from build123d import *

# Parameters (mm, degrees)
SKETCH_1_W             = 60
SKETCH_1_H             = 15
EXTRUDE_1_DEPTH        = 2
SKETCH_2_W             = 3
SKETCH_2_H             = 3
EXTRUDE_2_DEPTH        = 1
EXTRUDE_3_DEPTH        = 2
CUT_EXTRUDE_1_REACH    = 42.234
SKETCH_4_W             = 0.944409721
SKETCH_4_H             = 0.05
FILLET_1_R             = 0.1
FILLET_1_OF_MIRROR_2_R = 0.1
FILLET_2_R             = 0.2


# Read off the part's stored shape, not the designer's step: the mirror step
with BuildPart() as part:
    # Sketch 1 → Extrude 1 (new body)
    with BuildSketch(Plane.XY):
        Rectangle(SKETCH_1_W, SKETCH_1_H)
    extrude(amount=-EXTRUDE_1_DEPTH)

    # Sketch 2 → Extrude 2 (add)
    with BuildSketch(Plane.XY):
        with Locations((-7.5, 0)):
            Rectangle(SKETCH_2_W, SKETCH_2_H)
    extrude_2 = extrude(amount=EXTRUDE_2_DEPTH)

    # Sketch 3 → Extrude 3 (add, symmetric)
    with BuildSketch(Plane(origin=(0, 0, 0), x_dir=(1, 0, 0), z_dir=(0, 1, 0))):
        with BuildLine():
            Line((-9.45, -2.5), (-5.55, -2.5))
            Line((-5.55, -2.5), (-5.55, -1.555590279))
            ThreePointArc((-5.55, -1.555590279), (-5.719957697, -1.088161527), (-6, -0.677124344))
            Line((-6, -0.677124344), (-9, -0.677124344))
            ThreePointArc((-9, -0.677124344), (-9.280042303, -1.088161527), (-9.45, -1.555590279))
            Line((-9.45, -1.555590279), (-9.45, -2.5))
        make_face()
    extrude_3 = extrude(amount=EXTRUDE_3_DEPTH, both=True)

    # Sketch 4 → Cut-Extrude 1 (cut, up to next)
    with BuildSketch(Plane.ZY.offset(9.45), mode=Mode.PRIVATE) as cut_extrude_1_sk1:
        with BuildLine():
            Line((1.555590279, 1.95), (1.555590279, 2))
            Line((1.555590279, 2), (0.677124344, 2))
            Line((0.677124344, 2), (0.677124344, 1.5))
            ThreePointArc((0.677124344, 1.5), (1.088161527, 1.780042303), (1.555590279, 1.95))
        make_face()
    cut_extrude_1_tool1 = extrude(cut_extrude_1_sk1.sketch, amount=-CUT_EXTRUDE_1_REACH, mode=Mode.PRIVATE) & part.part
    # Sketch 4 → Cut-Extrude 1 (cut, up to next)
    with BuildSketch(Plane.ZY.offset(9.45), mode=Mode.PRIVATE) as cut_extrude_1_sk2:
        with Locations((2.02779514, 1.975)):
            Rectangle(SKETCH_4_W, SKETCH_4_H)
    cut_extrude_1_tool2 = extrude(cut_extrude_1_sk2.sketch, amount=-CUT_EXTRUDE_1_REACH, mode=Mode.PRIVATE) & part.part
    # Sketch 4 → Cut-Extrude 1 (cut, up to next)
    with BuildSketch(Plane.ZY.offset(9.45), mode=Mode.PRIVATE) as cut_extrude_1_sk3:
        with Locations((2.02779514, -1.975)):
            Rectangle(SKETCH_4_W, SKETCH_4_H)
    cut_extrude_1_tool3 = extrude(cut_extrude_1_sk3.sketch, amount=-CUT_EXTRUDE_1_REACH, mode=Mode.PRIVATE) & part.part
    # Sketch 4 → Cut-Extrude 1 (cut, up to next)
    with BuildSketch(Plane.ZY.offset(9.45), mode=Mode.PRIVATE) as cut_extrude_1_sk4:
        with BuildLine():
            Line((1.555590279, -2), (1.555590279, -1.95))
            ThreePointArc((1.555590279, -1.95), (1.088161527, -1.780042303), (0.677124344, -1.5))
            Line((0.677124344, -1.5), (0.677124344, -2))
            Line((0.677124344, -2), (1.555590279, -2))
        make_face()
    cut_extrude_1_tool4 = extrude(cut_extrude_1_sk4.sketch, amount=-CUT_EXTRUDE_1_REACH, mode=Mode.PRIVATE) & part.part
    cut_extrude_1_1 = cut_extrude_1_tool1.solids().sort_by_distance((-9.45, 1.849056, 0.974505))[0]
    add(cut_extrude_1_1, mode=Mode.SUBTRACT)
    cut_extrude_1_2 = cut_extrude_1_tool2.solids().sort_by_distance((-9.45, 1.975, 2.027795))[0]
    add(cut_extrude_1_2, mode=Mode.SUBTRACT)
    cut_extrude_1_3 = cut_extrude_1_tool3.solids().sort_by_distance((-9.45, -1.975, 2.027795))[0]
    add(cut_extrude_1_3, mode=Mode.SUBTRACT)
    cut_extrude_1_4 = cut_extrude_1_tool4.solids().sort_by_distance((-9.45, -1.849056, 0.974505))[0]
    add(cut_extrude_1_4, mode=Mode.SUBTRACT)
    cut_extrude_1 = cut_extrude_1_1 + cut_extrude_1_2 + cut_extrude_1_3 + cut_extrude_1_4  # Cut-Extrude 1 as one shape, for the pattern or mirror that repeats it

    # Fillet 1
    fillet_1_edges = [part.edges().sort_by_distance(p)[0] for p in [
        (-7.5, 1.95, 2.5),
        (-9.45, 0, 2.5),
        (-5.55, 0, 2.5),
        (-7.5, -1.95, 2.5),
    ]]
    fillet(fillet_1_edges, radius=FILLET_1_R)

    # Mirror 2: Extrude 2, Extrude 3, Cut-Extrude 1 across plane
    add(extrude_2.mirror(Plane(origin=(-15, 0, 0), x_dir=(0, 0, 1), z_dir=(1, 0, 0))))
    add(extrude_3.mirror(Plane(origin=(-15, 0, 0), x_dir=(0, 0, 1), z_dir=(1, 0, 0))))
    add(cut_extrude_1.mirror(Plane(origin=(-15, 0, 0), x_dir=(0, 0, 1), z_dir=(1, 0, 0))), mode=Mode.SUBTRACT)

    # Fillet 1 of Mirror 2
    fillet_1_of_mirror_2_edges = [part.edges().sort_by_distance(p)[0] for p in [
        (-22.5, 1.95, 2.5),
        (-20.55, 0, 2.5),
        (-24.45, 0, 2.5),
        (-22.5, -1.95, 2.5),
    ]]
    fillet(fillet_1_of_mirror_2_edges, radius=FILLET_1_OF_MIRROR_2_R)

    # Mirror 3: part across plane


with BuildPart() as part_1:
    add(part.part)
    add(part.part.mirror(Plane(origin=(0, 0, 0), x_dir=(0, 0, 1), z_dir=(1, 0, 0))))

    # Fillet 2
    fillet_2_edges = [part_1.edges().sort_by_distance(p)[0] for p in [
        (30, 0, -2),
        (0, 7.5, -2),
        (-30, 0, -2),
        (0, 7.5, 0),
        (30, 0, 0),
        (0, -7.5, 0),
        (-30, 0, 0),
        (0, -7.5, -2),
        (-30, 7.5, -1),
        (30, 7.5, -1),
        (30, -7.5, -1),
        (-30, -7.5, -1),
    ]]
    fillet(fillet_2_edges, radius=FILLET_2_R)


solid = part_1.part
Verification items for the finished model (mm, model axes). Coordinates: 2 decimals unless noted, no trailing zeros. Order: outer loops, then holes, each group sorted by start corner. A loop starts at its lowest first (then second) coordinate and runs counter-clockwise, first axis right, second up. Notation, with made-up numbers: M -4.5,44 L 13.5,44 A10 cw 13.5,50 Z; hole C 77,51 d5. An arc over 180 degrees is marked long. Return JSON: item names as keys, results as strings.
1) Cross-section at B-B, the plane y = 5.75. Record the boundary of the cut face in (x, z), and give its area (3 significant figures).
Answer list:
{"outline": "M -30,-1.8 A0.2 ccw -29.8,-2 L 29.8,-2 A0.2 ccw 30,-1.8 L 30,-0.2 A0.2 ccw 29.8,0 L -29.8,0 A0.2 ccw -30,-0.2 Z", "area": "120 mm2"}
2) Gauge pin test, flat ends, axial feed: pin 1 (0.7 mm diameter, centred on y = 0.5, z = 0.5, fed in from -X); pin 2 (0.7 mm diameter, centred on x = -8, z = 0.5, fed in from +Y); pin 3 (0.9 mm diameter, centred on y = 0, z = 2, fed in from +X). Record the tip position at first contact, or that the pin passes through.
Answer list:
{"pin 1": "x = -24.14", "pin 2": "y = 1.64", "pin 3": "x = 24.45"}
3) Thickness scan on L1, parallel to X at y = -6.25, z = -0.15; L2, parallel to Z at x = 23, y = 6.5; L3, parallel to Y at x = -3.5, z = -0.15. Record the ranges inside material, lowest first. Write a range as [from, to].
Answer list:
{"L1": "[-29.99, 29.99]", "L2": "[-2, 0]", "L3": "[-7.49, 7.49]"}
4) Cross-section at A-A, the plane x = -7.5. Record the boundary of the cut face in (y, z), and give its area (3 significant figures).
Answer list:
{"outline": "M -7.5,-1.8 A0.2 ccw -7.3,-2 L 7.3,-2 A0.2 ccw 7.5,-1.8 L 7.5,-0.2 A0.2 ccw 7.3,0 L 1.5,0 L 1.5,0.68 A2 ccw 1.95,1.56 L 1.95,2.4 A0.1 ccw 1.85,2.5 L -1.85,2.5 A0.1 ccw -1.95,2.4 L -1.95,1.56 A2 ccw -1.5,0.68 L -1.5,0 L -7.3,0 A0.2 ccw -7.5,-0.2 Z", "area": "38.8 mm2"}
